The model under review builds one solid part; all positions refer to its coordinate system, in mm. A direction names the side the tool comes from. Coordinates: 2 decimals unless noted, no trailing zeros. Write each loop counter-clockwise with the first axis right and the second up, starting at its lowest first coordinate (ties: lowest second). Pieces come first, ordered by that corner, then holes.
1) Add section A-A, the plane x = 0. State the section outline as (y, z) points, then the cut area to 3 significant figures.
2) Machinability: for faces 1 (the cylindrical face through (0.811, 1.282, 2.575)), 2 (the flat face through (0, 0, 3)), which of the approach directions +Z, -Z, +X, -X, +Y, -Y give a long, thin tool a straight path to every point of the face, cutting with its end or side? Answer none if there is none.
3) Add section B-B, the plane z = 0. State the section outline as (x, y) points, then the cut area to 3 significant figures.
4) For line 1 (X direction, y = 1.6, z = 0); line 2 (X direction, y = -1.1, z = 0); line 3 (Y direction, x = -4, z = 11), list the stretches that pass through material, from the lowest coordinate up.
5) Add section C-C, the plane y = 1.25. State the section outline as (x, z) points, then the cut area to 3 significant figures.
6) Add section D-D, the plane y = -0.75. State the section outline as (x, z) points.
7) For P1, Ø2, axis at x = -8, y = 2.5, coming from the -Z side; P2, Ø2, axis at x = 12, y = -0.5, coming from the -Z side; P3, Ø1.5, axis at y = 0, z = -10, coming from the +X side, all flat-tipped, find the tip position at first contact; note any pin that passes through.
from build123d import *

# Parameters (mm, degrees)
SKETCH1_R           = 16.5
SKETCH1_R_2         = 14.7
SKETCH1_R_3         = 2.7
BOSS_EXTRUDE1_DEPTH = 3
BOSS_EXTRUDE2_START = -3
SKETCH1_3_R         = 16.5
SKETCH1_3_R_2       = 14.7
BOSS_EXTRUDE2_DEPTH = 3
CHAMFER1_SIZE       = 0.4


with BuildPart() as part:
    # Sketch1 → Boss-Extrude1 (new body)
    # profile 1 of 2: a face of its own
    with BuildSketch(Plane(origin=(0, 0, 0), x_dir=(1, 0, 0), z_dir=(0, 1, 0))):
        with Locations(Location((0, 0, 0), (0, 0, 270))):
            Circle(SKETCH1_R)
        Circle(SKETCH1_R_2, mode=Mode.SUBTRACT)
    # profile 2 of 2: a face of its own
    with BuildSketch(Plane(origin=(0, 0, 0), x_dir=(1, 0, 0), z_dir=(0, 1, 0))):
        Circle(SKETCH1_R_2)
        with Locations(Location((0, 0, 0), (0, 0, 270))):
            Circle(SKETCH1_R_3, mode=Mode.SUBTRACT)
    extrude(amount=BOSS_EXTRUDE1_DEPTH)

    # Sketch1_3 → Boss-Extrude2 (add)
    with BuildSketch(Plane(origin=(0, 0, 0), x_dir=(1, 0, 0), z_dir=(0, 1, 0)).offset(BOSS_EXTRUDE2_START)):
        with Locations(Location((0, 0, 0), (0, 0, 270))):
            Circle(SKETCH1_3_R)
        with Locations(Location((0, 0, 0), (0, 0, 270))):
            Circle(SKETCH1_3_R_2, mode=Mode.SUBTRACT)
    extrude(amount=BOSS_EXTRUDE2_DEPTH)

    # Chamfer1
    chamfer1_edges = [part.edges().sort_by_distance(p)[0] for p in [
        (0, -3, -16.5),
        (0, -3, -14.7),
        (0, 3, -2.7),
        (0, 3, -16.5),
    ]]
    chamfer(chamfer1_edges, length=CHAMFER1_SIZE)


solid = part.part
Geometry results:
1. outline: (-3, -16.1) - (-2.6, -16.5) - (2.6, -16.5) - (3, -16.1) - (3, -3.1) - (2.6, -2.7) - (0, -2.7) - (0, -14.7) - (-2.6, -14.7) - (-3, -15.1) - close; (-3, 15.1) - (-2.6, 14.7) - (0, 14.7) - (0, 2.7) - (2.6, 2.7) - (3, 3.1) - (3, 16.1) - (2.6, 16.5) - (-2.6, 16.5) - (-3, 16.1) - close
1. area: 93.0 mm2
2. face 1: +Y, -Y
2. face 2: -Y
3. outline: (-16.5, -2.6) - (-16.1, -3) - (-15.1, -3) - (-14.7, -2.6) - (-14.7, 0) - (-2.7, 0) - (-2.7, 2.6) - (-3.1, 3) - (-16.1, 3) - (-16.5, 2.6) - close; (2.7, 0) - (14.7, 0) - (14.7, -2.6) - (15.1, -3) - (16.1, -3) - (16.5, -2.6) - (16.5, 2.6) - (16.1, 3) - (3.1, 3) - (2.7, 2.6) - close
3. area: 93.0 mm2
4. line 1: x = -16.5 to -2.7, 2.7 to 16.5
4. line 2: x = -16.5 to -14.7, 14.7 to 16.5
4. line 3: y = 0 to 3
5. outline: circle Ø33 at (0, 0); hole circle Ø5.4 at (0, 0)
5. area: 832 mm2
6. outline: circle Ø33 at (0, 0); hole circle Ø29.4 at (0, 0)
7. P1: stops at z = -14.94
7. P2: stops at z = -12.3
7. P3: stops at x = 13.66
